```python
from build123d import *

# Parameters (mm, degrees)
SKETCH_R    = 1
PAD_DEPTH   = 11
THICKNESS_T = -1.4


with BuildPart() as part:
    # Sketch → Pad (new body)
    with BuildSketch(Plane.XY):
        with BuildLine():
            Line((3, 0), (133, 0))
            ThreePointArc((133, 0), (135.12132, 0.87868), (136, 3))
            Line((136, 3), (136, 72))
            ThreePointArc((136, 72), (135.12132, 74.12132), (133, 75))
            Line((133, 75), (3, 75))
            ThreePointArc((3, 75), (0.87868, 74.12132), (0, 72))
            Line((0, 72), (0, 3))
            ThreePointArc((0, 3), (0.87868, 0.87868), (3, 0))
        make_face()
        with Locations((20, 67.486328)):
            Circle(SKETCH_R, mode=Mode.SUBTRACT)
        with Locations((43, 70.986328)):
            Circle(SKETCH_R, mode=Mode.SUBTRACT)
        with Locations((93, 71)):
            Circle(SKETCH_R, mode=Mode.SUBTRACT)
        with Locations((4, 4)):
            Circle(SKETCH_R, mode=Mode.SUBTRACT)
        with BuildLine():
            Line((104.5, 68), (104.5, 3.221195))
            ThreePointArc((104.5, 3.221195), (104.792893, 2.514089), (105.5, 2.221195))
            Line((105.5, 2.221195), (133.5, 2.221195))
            ThreePointArc((133.5, 2.221195), (134.207107, 2.514089), (134.5, 3.221195))
            Line((134.5, 3.221195), (134.5, 68))
            ThreePointArc((134.5, 68), (134.207107, 68.707107), (133.5, 69))
            Line((133.5, 69), (105.5, 69))
            ThreePointArc((105.5, 69), (104.792893, 68.707107), (104.5, 68))
        make_face(mode=Mode.SUBTRACT)
    extrude(amount=PAD_DEPTH)

    # Thickness
    thickness_openings = [part.faces().sort_by_distance(p)[0] for p in [
        (55.431253, 37.938308, 11),
        (104.5, 35.610598, 5.5),
        (104.792893, 68.707107, 5.5),
        (119.5, 69, 5.5),
        (134.207107, 68.707107, 5.5),
        (134.5, 35.610598, 5.5),
        (119.5, 2.221195, 5.5),
        (134.207107, 2.514089, 5.5),
        (104.792893, 2.514089, 5.5),
        (92, 71, 5.5),
        (42, 70.986328, 5.5),
        (19, 67.486328, 5.5),
        (3, 4, 5.5),
    ]]
    offset(amount=THICKNESS_T, openings=thickness_openings)


solid = part.part
```
Source: CAD feature listing. Evaluate the final solid. Frame: model axes, mm. A direction names the side the tool comes from. Round coordinates to 2 decimals unless told otherwise and drop trailing zeros. Loops run counter-clockwise (first coordinate to the right, second up) from the corner with the lowest first, then second, coordinate; pieces in that order, holes last. Notation, with made-up numbers: M -30,30.5 L -5,30.5 A20 cw -5,57.5 Z; hole C -23.5,22 d11. An arc over 180 degrees is marked long. Use a Markdown table: item, result. Add a question column.
1. Mould query, pull axis Y, two halves, no side actions, for faces 3 (the flat face through (52, 38, 1.4)), 4 (the flat face through (69, 73.6, 6)), 5 (the cylindrical face through (135.1, 0.86, 5.42)), 6 (the cylindrical face through (135.14, 74.1, 5.42)). Classes: pulls with the +Y half, pulls with the -Y half, needs draft (parallel to the pull), parting line crosses it, or undercut.
2. Line query: line 1 (X direction, y = 71, z = 0.6); line 2 (Y direction, x = 20, z = 0.4); line 3 (Y direction, x = 39.5, z = 7.5). Output: solid intervals per line, ascending.
3. Section query B-B on x = 81. Return the cut outline in (y, z), then the cut area to 3 significant figures.
4. Contact query for flat-ended pins moving along their axis: P1, Ø1, axis at x = 48, y = 66, coming from the -Z side; P2, Ø3, axis at x = 43, y = 70.99, coming from the +Z side; P3, Ø1.6, axis at x = 4, y = 4, coming from the -Z side. Output: stop coordinate, or through.
5. Section query A-A on y = 16. Return the cut outline in (x, z).
6. Section query C-C on z = 6.25. Return the cut outline in (x, y), then the cut area to 3 significant figures.
7. Reachability of faces 1 (the flat face through (67, 0, 5)), 2 (the flat face through (134.6, 37, 6)) from +Z, -Z, +X, -X, +Y, -Y: full face, straight path, thin tool, end or side. Return the list, or none.
Reported:
| question | item | result |
|---|---|---|
| 1 | face 3 | undercut |
| 1 | face 4 | undercut |
| 1 | face 5 | pulls with the -Y half |
| 1 | face 6 | pulls with the +Y half |
| 2 | line 1 | x = 0 to 42, 44 to 92, 94 to 136 |
| 2 | line 2 | y = 0 to 66.49, 68.49 to 75 |
| 2 | line 3 | y = 0 to 1.4, 73.6 to 75 |
| 3 | outline | M 0,0 L 75,0 L 75,11 L 73.6,11 L 73.6,1.4 L 1.4,1.4 L 1.4,11 L 0,11 Z |
| 3 | area | 132 mm² |
| 4 | P1 | stops at z = 0 |
| 4 | P2 | stops at z = 1.4 |
| 4 | P3 | passes through |
| 5 | outline | M 0,0 L 104.5,0 L 104.5,1.4 L 1.4,1.4 L 1.4,11 L 0,11 Z; M 134.5,0 L 136,0 L 136,11 L 134.6,11 L 134.6,1.4 L 134.5,1.4 Z |
| 6 | outline | M 0,3 A3 ccw 3,0 L 133,0 A3 ccw 136,3 L 136,72 A3 ccw 133,75 L 3,75 A3 ccw 0,72 Z; hole M 1.4,3 A1.6 ccw 3,1.4 L 133,1.4 A1.6 ccw 134.6,3 L 134.6,72 A1.6 ccw 133,73.6 L 3,73.6 A1.6 ccw 1.4,72 Z |
| 6 | area | 577 mm² |
| 7 | face 1 | +Z, -Z, +X, -X, -Y |
| 7 | face 2 | +Z |
